```python
from build123d import *

# Parameters (mm, degrees)
SKETCH1_R           = 2.413
SKETCH1_R_2         = 3.429
BOSS_EXTRUDE1_DEPTH = 5.08
SKETCH2_R           = 5.715
SKETCH2_R_2         = 2.413
BOSS_EXTRUDE2_DEPTH = 25.4


with BuildPart() as part:
    # Sketch1 → Boss-Extrude1 (new body)
    with BuildSketch(Plane.XY):
        with BuildLine():
            ThreePointArc((21.211318458, -5.238895267), (29.21, 0), (21.211318458, 5.238895267))
            add(Edge.make_bspline(
                [(21.211318458, 5.238895267), (0, 11.083329031), (-21.211318458, 5.238895267)],
                knots=[3.899659671, 3.899659671, 3.899659671, 5.525118289, 5.525118289, 5.525118289], degree=2, weights=[1, 0.687519064, 1]))
            ThreePointArc((-21.211318458, 5.238895267), (-29.21, 0), (-21.211318458, -5.238895267))
            add(Edge.make_bspline(
                [(-21.211318458, -5.238895267), (0, -11.083329031), (21.211318458, -5.238895267)],
                knots=[0.758067018, 0.758067018, 0.758067018, 2.383525636, 2.383525636, 2.383525636], degree=2, weights=[1, 0.687519064, 1]))
        make_face()
        with Locations((-23.495, 0)):
            Circle(SKETCH1_R, mode=Mode.SUBTRACT)
        Circle(SKETCH1_R_2, mode=Mode.SUBTRACT)
        with Locations((23.495, 0)):
            Circle(SKETCH1_R, mode=Mode.SUBTRACT)
    extrude(amount=BOSS_EXTRUDE1_DEPTH)

    # Sketch2 → Boss-Extrude2 (add)
    with BuildSketch(Plane(origin=(0, 0, 0), x_dir=(-1, 0, 0), z_dir=(0, 0, -1))):
        with Locations((-23.495, 0)):
            Circle(SKETCH2_R)
        with Locations((-23.495, 0)):
            Circle(SKETCH2_R_2, mode=Mode.SUBTRACT)
        with Locations((23.495, 0)):
            Circle(SKETCH2_R)
        with Locations((23.495, 0)):
            Circle(SKETCH2_R_2, mode=Mode.SUBTRACT)
    extrude(amount=BOSS_EXTRUDE2_DEPTH)


solid = part.part
```
CAD build for the part. Positions are in the model's coordinates, mm. Coordinates: 2 decimals unless noted, no trailing zeros. Order: outer loops, then holes, each group sorted by start corner. A loop starts at its lowest first (then second) coordinate and runs counter-clockwise, first axis right, second up. Notation, with made-up numbers: (12.5, -4) -> (28.5, -4) arc R29 cw to (28.5, 32) -> close; hole circle Ø2 at (-29, 50.25). An arc over 180 degrees is marked (long way). Use one line per item in the form item = value. Start each with the question number.
1) Drill centre lines: L1, parallel to X at y = 0, z = -12.5; L2, parallel to Y at x = 24.5, z = -19; L3, parallel to Z at x = 4.5, y = 0.5. Where is each one in solid material? Low to high. Write a range as [from, to].
2) Band-saw the part on D-D on y = -4.5. Give the cut face in (x, z).
3) Band-saw the part on B-B on z = -10.5. Give the cut face in (x, y) (3 decimals).
4) Band-saw the part on A-A on y = 0. Give the cut face in (x, z).
5) Band-saw the part on C-C on x = -24. Give the cut face in (y, z).
6) Pull direction X, two halves, no side cores. Call faces 1 (the cylindrical face through (-28.378, 2.97, -9.947)), 2 (the flat face through (-24.7, -2.5, -25.4)), 3 (the cylindrical face through (-0.74, -3.35, 2.5)): +X half, -X half, draft (parallel to the pull), parting line (faces both ways), or undercut.
7) Drop flat-ended pins along their axis: pin 1 (1.5 mm diameter, centred on y = -2, z = -11.5, fed in from +X); pin 2 (2 mm diameter, centred on x = 1.5, y = -2, fed in from -Z); pin 3 (10 mm diameter, centred on x = -5.5, z = 0.5, fed in from -Y); pin 4 (4.5 mm diameter, centred on x = -23.495, y = 0, fed in from +Z). Give the stop position or say it passes through.
Entries:
q1.L1 = [-29.21, -25.91], [-21.08, -17.78], [17.78, 21.08], [25.91, 29.21]
q1.L2 = [-5.63, -2.19], [2.19, 5.63]
q1.L3 = [0, 5.08]
q2.outline = (-27.02, -25.4) -> (-19.97, -25.4) -> (-19.97, 0) -> (19.97, 0) -> (19.97, -25.4) -> (27.02, -25.4) -> (27.02, 5.08) -> (-27.02, 5.08) -> close
q3.outline = circle Ø11.43 at (-23.495, 0); circle Ø11.43 at (23.495, 0); hole circle Ø4.826 at (-23.495, 0); hole circle Ø4.826 at (23.495, 0)
q4.outline = (-29.21, -25.4) -> (-25.91, -25.4) -> (-25.91, 5.08) -> (-29.21, 5.08) -> close; (-21.08, -25.4) -> (-17.78, -25.4) -> (-17.78, 0) -> (-3.43, 0) -> (-3.43, 5.08) -> (-21.08, 5.08) -> close; (3.43, 0) -> (17.78, 0) -> (17.78, -25.4) -> (21.08, -25.4) -> (21.08, 5.08) -> (3.43, 5.08) -> close; (25.91, -25.4) -> (29.21, -25.4) -> (29.21, 5.08) -> (25.91, 5.08) -> close
q5.outline = (-5.69, -25.4) -> (-2.36, -25.4) -> (-2.36, 5.08) -> (-5.69, 5.08) -> close; (2.36, -25.4) -> (5.69, -25.4) -> (5.69, 5.08) -> (2.36, 5.08) -> close
q6.face_1 = undercut
q6.face_2 = draft
q6.face_3 = undercut
q7.pin_1 = 29.07
q7.pin_2 = 0
q7.pin_3 = -7.62
q7.pin_4 = through
